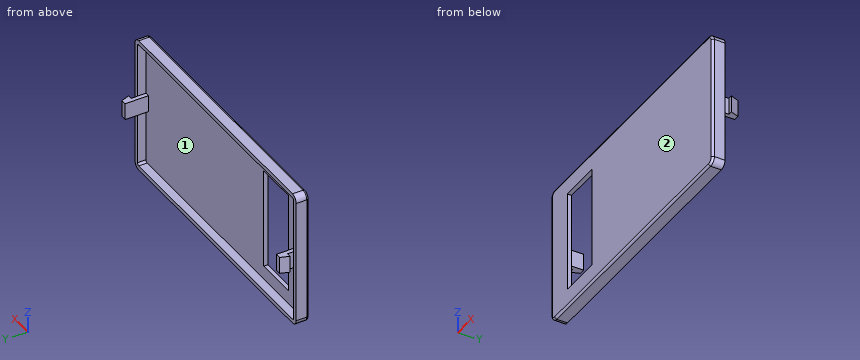
from build123d import *

# Parameters (mm, degrees)
SKETCH_1_W                  = 130
SKETCH_1_H                  = 65
EXTRUDE_1_DEPTH             = 6
SKETCH_2_W                  = 126
SKETCH_2_H                  = 61
CUT_EXTRUDE_1_DEPTH         = 4
FILLET_1_R                  = 1
SKETCH_9_W                  = 20
SKETCH_9_H                  = 48
CUT_EXTRUDE_3_DEPTH         = 2
SKETCH_6_W                  = 2
SKETCH_6_H                  = 8
EXTRUDE_2_DEPTH             = 11
SKETCH_12_W                 = 8
SKETCH_12_H                 = 4
EXTRUDE_4_DEPTH             = 2
CHAMFER_2_SIZE2             = 4
CHAMFER_2_SIZE              = 1.455880937
CHAMFER_2_OF_MIRROR_2_SIZE2 = 1.455880937
CHAMFER_2_OF_MIRROR_2_SIZE  = 4
FILLET_2_R                  = 1
FILLET_3_R                  = 3


# Some blends are built 0.0001 mm under size
with BuildPart() as part:
    # Эскиз1 → Бобышка-Вытянуть1 (new body)
    with BuildSketch(Plane(origin=(0, 0, 0), x_dir=(1, 0, 0), z_dir=(0, 1, 0))):
        Rectangle(SKETCH_1_W, SKETCH_1_H)
    extrude(amount=EXTRUDE_1_DEPTH)

    # Эскиз2 → Вырез-Вытянуть1 (cut)
    with BuildSketch(Plane(origin=(0, 6, 0), x_dir=(1, 0, 0), z_dir=(0, 1, 0))):
        Rectangle(SKETCH_2_W, SKETCH_2_H)
    extrude(amount=-CUT_EXTRUDE_1_DEPTH, mode=Mode.SUBTRACT)

    # Скругление1
    fillet_1_edges = [part.edges().sort_by_distance(p)[0] for p in [
        (0, 0, 32.5),
        (-65, 0, 0),
        (0, 0, -32.5),
        (65, 0, 0),
    ]]
    fillet(fillet_1_edges, radius=FILLET_1_R)

    # Эскиз9 → Вырез-Вытянуть3 (cut)
    with BuildSketch(Plane.XZ):
        with Locations((-42, 0)):
            Rectangle(SKETCH_9_W, SKETCH_9_H)
    extrude(amount=-CUT_EXTRUDE_3_DEPTH, mode=Mode.SUBTRACT)

    # Эскиз6 → Бобышка-Вытянуть2 (add)
    with BuildSketch(Plane(origin=(0, 2, 0), x_dir=(1, 0, 0), z_dir=(0, 1, 0))):
        with Locations((62, 0)):
            Rectangle(SKETCH_6_W, SKETCH_6_H)
    extrude_2 = extrude(amount=EXTRUDE_2_DEPTH)

    # Эскиз12 → Бобышка-Вытянуть4 (add)
    with BuildSketch(Plane(origin=(63, 0, 0), x_dir=(0, 0, -1), z_dir=(1, 0, 0))):
        with Locations((0, 11)):
            Rectangle(SKETCH_12_W, SKETCH_12_H)
    extrude_4 = extrude(amount=EXTRUDE_4_DEPTH)

    # Фаска2
    chamfer_2_edges = [part.edges().sort_by_distance(p)[0] for p in [
        (65, 13, 0),
    ]]
    chamfer_2_side = [part.faces().sort_by_distance(p)[0] for p in [
        (64.970882381, 13, 0),
    ]]
    chamfer(chamfer_2_edges, length=CHAMFER_2_SIZE - 0.0001, length2=CHAMFER_2_SIZE2 - 0.0001, reference=chamfer_2_side[0])  # a hair under: the kernel refuses the full size

    # Зеркальное отражение2: Бобышка-Вытянуть2, Бобышка-Вытянуть4 across plane
    add(extrude_2.mirror(Plane(origin=(0, 0, 0), x_dir=(0, 0, 1), z_dir=(1, 0, 0))))
    add(extrude_4.mirror(Plane(origin=(0, 0, 0), x_dir=(0, 0, 1), z_dir=(1, 0, 0))))

    # Фаска2 of Зеркальное отражение2
    chamfer_2_of_mirror_2_edges = [part.edges().sort_by_distance(p)[0] for p in [
        (-65, 13, 0),
    ]]
    chamfer_2_of_mirror_2_side = [part.faces().sort_by_distance(p)[0] for p in [
        (-65, 12.970882381, 0),
    ]]
    chamfer(chamfer_2_of_mirror_2_edges, length=CHAMFER_2_OF_MIRROR_2_SIZE - 0.0001, length2=CHAMFER_2_OF_MIRROR_2_SIZE2 - 0.0001, reference=chamfer_2_of_mirror_2_side[0])  # a hair under: the kernel refuses the full size

    # Скругление2
    fillet_2_edges = [part.edges().sort_by_distance(p)[0] for p in [
        (63, 4, -30.5),
        (63, 4, 30.5),
        (-63, 4, 30.5),
        (-63, 4, -30.5),
    ]]
    fillet(fillet_2_edges, radius=FILLET_2_R)

    # Скругление3
    # the kernel refuses this fillet: 3 mm, written as the material it takes off along each edge
    with BuildSketch(Plane(origin=(-62, 0, 29.5), x_dir=(0, 0, 1), z_dir=(1, 0, 0))) as fillet_3_piece_1:
        with BuildLine():
            CenterArc((2, -1), 1, 0, 90)
            Line((3, -1), (3, 0))
            Line((3, 0), (2, 0))
        make_face()
    revolve(axis=Axis((-62, 0, 29.5), (0, -1, 0)), revolution_arc=90, mode=Mode.SUBTRACT)
    with BuildSketch(Plane(origin=(-62, 0, -29.5), x_dir=(-1, 0, 0), z_dir=(0, 0, 1))) as fillet_3_piece_2:
        with BuildLine():
            CenterArc((2, -1), 1, 0, 90)
            Line((3, -1), (3, 0))
            Line((3, 0), (2, 0))
        make_face()
    revolve(axis=Axis((-62, 0, -29.5), (0, -1, 0)), revolution_arc=90, mode=Mode.SUBTRACT)
    with BuildSketch(Plane(origin=(62, 0, 29.5), x_dir=(1, 0, 0), z_dir=(0, 0, -1))) as fillet_3_piece_3:
        with BuildLine():
            CenterArc((2, -1), 1, 0, 90)
            Line((3, -1), (3, 0))
            Line((3, 0), (2, 0))
        make_face()
    revolve(axis=Axis((62, 0, 29.5), (0, -1, 0)), revolution_arc=90, mode=Mode.SUBTRACT)
    with BuildSketch(Plane(origin=(62, 0, -29.5), x_dir=(0, 0, -1), z_dir=(-1, 0, 0))) as fillet_3_piece_4:
        with BuildLine():
            CenterArc((2, -1), 1, 0, 90)
            Line((3, -1), (3, 0))
            Line((3, 0), (2, 0))
        make_face()
    revolve(axis=Axis((62, 0, -29.5), (0, -1, 0)), revolution_arc=90, mode=Mode.SUBTRACT)
    with BuildSketch(Plane(origin=(65, 0, 32.5), x_dir=(-1, 0, 0), z_dir=(0, 1, 0)), Plane(origin=(65, 0, -32.5), x_dir=(0, 0, 1), z_dir=(0, 1, 0))) as fillet_3_piece_5:
        with BuildLine():
            CenterArc((FILLET_3_R, -FILLET_3_R), FILLET_3_R, 90, 90)
            Line((0, -FILLET_3_R), (0, 0))
            Line((0, 0), (FILLET_3_R, 0))
        make_face()
    extrude(amount=13.5, mode=Mode.SUBTRACT)
    with BuildSketch(Plane(origin=(-65, 0, 32.5), x_dir=(1, 0, 0), z_dir=(0, 1, 0)), Plane(origin=(-65, 0, -32.5), x_dir=(0, 0, 1), z_dir=(0, 1, 0))) as fillet_3_piece_6:
        with BuildLine():
            CenterArc((FILLET_3_R, FILLET_3_R), FILLET_3_R, 180, 90)
            Line((0, FILLET_3_R), (0, 0))
            Line((0, 0), (FILLET_3_R, 0))
        make_face()
    extrude(amount=13.5, mode=Mode.SUBTRACT)


solid = part.part
Can you work these out from the model? Positions are in its coordinate system, mm. Face numbers are marked on the shaded views. Coordinates: 2 decimals unless noted, no trailing zeros. Loops run counter-clockwise (first coordinate to the right, second up) from the corner with the lowest first, then second, coordinate; pieces in that order, holes last. Notation, with made-up numbers: M 79,73 L 94,73 A12 cw 94,91 Z; hole C -29.5,3.5 d10. An arc over 180 degrees is marked long. Return JSON: item names as keys, results as strings. Group by question number.
Item 1: Imagine slicing it at A-A (x = -34). Please give me the cut outline in (y, z), and give its area (3 significant figures).
Item 2: I'm going to push flat-ended pins straight in: pin 1 Ø10 at (x, z) = (36, 19) entering from +Y; pin 2 Ø2 at (y, z) = (0.5, 10) entering from +X; pin 3 Ø1.5 at (y, z) = (7, -1) entering from +X; pin 4 Ø0.6 at (x, z) = (-64.5, -1.5) entering from -Y. Where does each tip first touch, or does it pass through?
Item 3: If I drill on L1, parallel to Z at x = 37.5, y = 2.75; L2, parallel to X at y = 2.75, z = -0.5; L3, parallel to Y at x = 20, z = -8.5, over which ranges is the centre line in solid material (lowest first)? Write a range as from..to.
Item 4: Thinking about a two-plate mould opening in X: for the marked faces 1 and 2, which applies, released by +X, released by -X, zero draft, split by the parting line, or undercut?
Item 5: Imagine slicing it at B-B (y = 3.25). Please give me the cut outline in (x, z), and give its area (3 significant figures).
Item 6: Imagine slicing it at C-C (z = -22.5). Please give me the cut outline in (x, y), and give its area (3 significant figures).
Item 7: Imagine slicing it at D-D (x = 42). Please give me the cut outline in (y, z).
Verdict:
{
 "1": {"outline": "M 0,-31.5 A1 ccw 1,-32.5 L 6,-32.5 L 6,-30.5 L 2,-30.5 L 2,-24 L 0,-24 Z; M 0,24 L 2,24 L 2,30.5 L 6,30.5 L 6,32.5 L 1,32.5 A1 ccw 0,31.5 Z", "area": "49.6 mm^2"},
 "2": {"pin 1": "stops at y = 2", "pin 2": "stops at x = 65", "pin 3": "stops at x = 63", "pin 4": "stops at y = 0.02"},
 "3": {"L1": "z = -32.5..-30.5, 30.5..32.5", "L2": "x = -65..-61, 61..65", "L3": "y = 0..2"},
 "4": {"face 1": "undercut", "face 2": "zero draft"},
 "5": {"outline": "M -65,-29.5 A3 ccw -62,-32.5 L 62,-32.5 A3 ccw 65,-29.5 L 65,29.5 A3 ccw 62,32.5 L -62,32.5 A3 ccw -65,29.5 Z; hole M -63,-29.5 A1 ccw -62,-30.5 L 62,-30.5 A1 ccw 63,-29.5 L 63,-4 L 61,-4 L 61,4 L 63,4 L 63,29.5 A1 ccw 62,30.5 L -62,30.5 A1 ccw -63,29.5 L -63,4 L -61,4 L -61,-4 L -63,-4 Z", "area": "789 mm^2"},
 "6": {"outline": "M -65,1 A1 ccw -64,0 L -52,0 L -52,2 L -63,2 L -63,6 L -65,6 Z; M -32,0 L 64,0 A1 ccw 65,1 L 65,6 L 63,6 L 63,2 L -32,2 Z", "area": "236 mm^2"},
 "7": {"outline": "M 0,-31.5 A1 ccw 1,-32.5 L 6,-32.5 L 6,-30.5 L 2,-30.5 L 2,30.5 L 6,30.5 L 6,32.5 L 1,32.5 A1 ccw 0,31.5 Z"}
}
